```python
from build123d import *

# Parameters (mm, degrees)
SKETCH1_W           = 107.95
SKETCH1_H           = 7.62
BOSS_EXTRUDE1_DEPTH = 5.08
SKETCH2_W           = 7.62
SKETCH2_H           = 7.62
BOSS_EXTRUDE2_DEPTH = 33.02
SKETCH3_R           = 1.778
CUT_EXTRUDE1_DEPTH  = 7.62
SKETCH4_R           = 2.286
CUT_EXTRUDE2_DEPTH  = 7.62
SKETCH5_R           = 2.1717
CUT_EXTRUDE3_DEPTH  = 5.08


with BuildPart() as part:
    # Sketch1 → Boss-Extrude1 (new body)
    with BuildSketch(Plane(origin=(0, 0, 0), x_dir=(1, 0, 0), z_dir=(0, 1, 0))):
        with Locations((-53.975, -10.454877129)):
            Rectangle(SKETCH1_W, SKETCH1_H)
    extrude(amount=BOSS_EXTRUDE1_DEPTH)

    # Sketch2 → Boss-Extrude2 (add)
    with BuildSketch(Plane(origin=(0, 5.08, 0), x_dir=(1, 0, 0), z_dir=(0, 1, 0))):
        with Locations((-104.14, -10.454877129)):
            Rectangle(SKETCH2_W, SKETCH2_H)
        with Locations((-3.81, -10.454877129)):
            Rectangle(SKETCH2_W, SKETCH2_H)
    extrude(amount=BOSS_EXTRUDE2_DEPTH)

    # Sketch3 → Cut-Extrude1 (cut)
    with BuildSketch(Plane(origin=(-100.33, 0, 0), x_dir=(0, 0, -1), z_dir=(1, 0, 0))):
        with Locations((-10.454877129, 33.02)):
            Circle(SKETCH3_R)
        with Locations((-10.454877129, 10.795)):
            Circle(SKETCH3_R)
    extrude(amount=-CUT_EXTRUDE1_DEPTH, mode=Mode.SUBTRACT)

    # Sketch4 → Cut-Extrude2 (cut)
    with BuildSketch(Plane.ZY.offset(7.62)):
        with Locations((10.454877129, 21.9075)):
            Circle(SKETCH4_R)
    extrude(amount=-CUT_EXTRUDE2_DEPTH, mode=Mode.SUBTRACT)

    # Sketch5 → Cut-Extrude3 (cut)
    with BuildSketch(Plane(origin=(0, 5.08, 0), x_dir=(1, 0, 0), z_dir=(0, 1, 0))):
        with Locations(Location((-87.63, -10.454877129, 0), (0, 0, 270))):
            Circle(SKETCH5_R)
        with Locations(Location((-68.58, -10.454877129, 0), (0, 0, 270))):
            Circle(SKETCH5_R)
        with Locations(Location((-49.53, -10.454877129, 0), (0, 0, 270))):
            Circle(SKETCH5_R)
        with Locations(Location((-30.48, -10.454877129, 0), (0, 0, 270))):
            Circle(SKETCH5_R)
    extrude(amount=-CUT_EXTRUDE3_DEPTH, mode=Mode.SUBTRACT)


solid = part.part
```
Can you work these out from the model? Positions are in its coordinate system, mm. A direction names the side the tool comes from. Coordinates: 2 decimals unless noted, no trailing zeros. Loops run counter-clockwise (first coordinate to the right, second up) from the corner with the lowest first, then second, coordinate; pieces in that order, holes last. Notation, with made-up numbers: (-16, 34.25) - (10, 34.25) arc R19 ccw to (10, 63.25) - close; hole circle Ø7 at (-7.75, 49). An arc over 180 degrees is marked (long way). Answer as CSV lines item,"result". Start each with the question number.
1) Suppose I cut it at A-A (y = 33.02). Please give me the cut outline in (x, z), plus the area to 3 significant figures.
2) I need wall thicknesses on line 1 (X direction, y = 14, z = 8.5); line 2 (X direction, y = 4.5, z = 9.5); line 3 (Y direction, x = -85, z = 11.75). Which ranges of each line are inside material? Lowest first, please. Write a range as from..to.
3) Suppose I cut it at C-C (y = 6). Please give me the cut outline in (x, z), plus the area to 3 significant figures.
4) Suppose I cut it at B-B (x = -49.53). Please give me the cut outline in (y, z).
5) Thinking about a two-plate mould opening in Y: for faces 1 (the cylindrical face through (-104.09, 9.22, 9.63)), 2 (the flat face through (-55, 0, 10)), 3 (the flat face through (-54.2, 4.8, 6.645)), 4 (the flat face through (-4, 38.1, 10)), which applies, pulls with the +Y half, pulls with the -Y half, needs draft (parallel to the pull), parting line crosses it, or undercut?
6) Which directions (+Z, -Z, +X, -X, +Y, -Y) give clear straight access to the entire face, cutting with the end or side of a thin tool? Please do faces 5 (the cylindrical face through (-70.7, 2.58, 9.98)), 6 (the flat face through (-100.33, 21, 11)), 7 (the cylindrical face through (-104.09, 34.52, 9.5)), 8 (the cylindrical face through (-3.86, 19.88, 11.51)), 9 (the flat face through (0, 19, 11)).
7) For pin 1 (1.5 mm diameter, centred on x = -57, z = 10.5, fed in from +Y), with a flat end and sliding along its axis, tell me the tip position at first contact or that it passes through.
Check result:
1,outline,"(-107.95, 6.64) - (-100.33, 6.64) - (-100.33, 8.68) - (-107.95, 8.68) - close; (-107.95, 12.23) - (-100.33, 12.23) - (-100.33, 14.26) - (-107.95, 14.26) - close; (-7.62, 6.64) - (0, 6.64) - (0, 14.26) - (-7.62, 14.26) - close"
1,area,"89.0 mm²"
2,line 1,"x = -107.95..-100.33, -7.62..0"
2,line 2,"x = -107.95..-89.58, -85.68..-70.53, -66.63..-51.48, -47.58..-32.43, -28.53..0"
2,line 3,"y = 0..5.08"
3,outline,"(-107.95, 6.64) - (-100.33, 6.64) - (-100.33, 14.26) - (-107.95, 14.26) - close; (-7.62, 6.64) - (0, 6.64) - (0, 14.26) - (-7.62, 14.26) - close"
3,area,"116 mm²"
4,outline,"(0, 6.64) - (5.08, 6.64) - (5.08, 8.28) - (0, 8.28) - close; (0, 12.63) - (5.08, 12.63) - (5.08, 14.26) - (0, 14.26) - close"
5,face 1,"undercut"
5,face 2,"pulls with the -Y half"
5,face 3,"needs draft"
5,face 4,"pulls with the +Y half"
6,face 5,"+Y, -Y"
6,face 6,"+Z, -Z, +Y"
6,face 7,"-X"
6,face 8,"+X"
6,face 9,"+Z, -Z, +X, +Y, -Y"
7,pin 1,"stops at y = 5.08"
